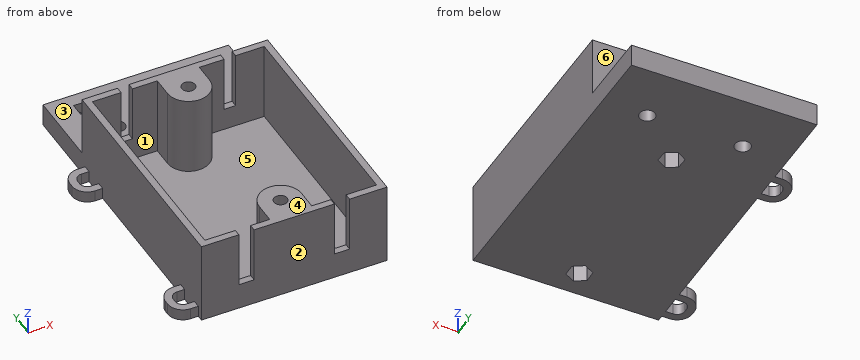
```python
from build123d import *

# Parameters (mm, degrees)
F0_W      = 48.6
F0_H      = 61.2
F1_DEPTH  = 22
F0_R      = 1.75
F2_DEPTH  = 22
F3_DEPTH  = 1
F0_H_2    = 20
F0_R_2    = 2.05
F4_DEPTH  = 6
F5_W      = 3
F5_H      = 1.8
F5_W_2    = 4
F6_DEPTH  = 15
F8_DEPTH  = 7
F9_DEPTH  = 3.5
F11_DEPTH = 5.2
F12_DEPTH = 5
F14_DEPTH = 3


with BuildPart() as f1:
    # F0 (on Top) → F1 (new body)
    with BuildSketch(Plane.XY):
        Rectangle(F0_W, F0_H)
        Polygon((22.5, 28.8), (22.5, -28.8), (5.5, -28.8), (-5.5, -28.8), (-22.5, -28.8), (-22.5, 28.8), (-5.5, 28.8), (5.5, 28.8), align=None, mode=Mode.SUBTRACT)
    extrude(amount=F1_DEPTH)

    # F0 (on Top) → F2 (join)
    with BuildSketch(Plane.XY):
        with BuildLine():
            Line((-5.5, -28.8), (5.5, -28.8))
            Line((5.5, -28.8), (5.5, -23.6))
            ThreePointArc((5.5, -23.6), (0, -18.1), (-5.5, -23.6))
            Line((-5.5, -23.6), (-5.5, -28.8))
        make_face()
        with Locations((0, -23.6)):
            Circle(F0_R, mode=Mode.SUBTRACT)
        with BuildLine():
            Line((5.5, 23.6), (5.5, 28.8))
            Line((5.5, 28.8), (-5.5, 28.8))
            Line((-5.5, 28.8), (-5.5, 23.6))
            ThreePointArc((-5.5, 23.6), (0, 18.1), (5.5, 23.6))
        make_face()
        with Locations((0, 23.6)):
            Circle(F0_R, mode=Mode.SUBTRACT)
    extrude(amount=F2_DEPTH)

    # F0 (on Top) → F3 (join)
    with BuildSketch(Plane.XY):
        with BuildLine():
            Line((5.5, -28.8), (22.5, -28.8))
            Line((22.5, -28.8), (22.5, 28.8))
            Line((22.5, 28.8), (5.5, 28.8))
            Line((5.5, 28.8), (5.5, 23.6))
            ThreePointArc((5.5, 23.6), (0, 18.1), (-5.5, 23.6))
            Line((-5.5, 23.6), (-5.5, 28.8))
            Line((-5.5, 28.8), (-22.5, 28.8))
            Line((-22.5, 28.8), (-22.5, -28.8))
            Line((-22.5, -28.8), (-5.5, -28.8))
            Line((-5.5, -28.8), (-5.5, -23.6))
            ThreePointArc((-5.5, -23.6), (0, -18.1), (5.5, -23.6))
            Line((5.5, -23.6), (5.5, -28.8))
        make_face()
    extrude(amount=F3_DEPTH)

    # F0 (on Top) → F4 (join)
    with BuildSketch(Plane.XY):
        with Locations((0, 40.6)):
            Rectangle(F0_W, F0_H_2)
        with Locations((-12.5, 35.6)):
            Circle(F0_R_2, mode=Mode.SUBTRACT)
        with Locations((12.5, 35.6)):
            Circle(F0_R_2, mode=Mode.SUBTRACT)
    extrude(amount=F4_DEPTH)

    # F5 (on face) → F6 (cut)
    with BuildSketch(Plane.XY.offset(22)):
        with Locations((-13.5, 29.7)):
            Rectangle(F5_W, F5_H)
        with Locations((13.5, 29.7)):
            Rectangle(F5_W, F5_H)
        with Locations((-12.5, -29.7)):
            Rectangle(F5_W_2, F5_H)
        with Locations((12.5, -29.7)):
            Rectangle(F5_W_2, F5_H)
    extrude(amount=-F6_DEPTH, mode=Mode.SUBTRACT)

    # F7 (on face) → F8 (cut)
    with BuildSketch(Plane(origin=(0, 50.6, 0), x_dir=(-1, 0, 0), z_dir=(0, 1, 0))):
        with BuildLine():
            Line((11, 6), (8.9152066989, 6))
            ThreePointArc((8.9152066989, 6), (13.5, 2.3074175964), (18.0847933011, 6))
            Line((18.0847933011, 6), (16, 6))
            ThreePointArc((16, 6), (13.5, 4.3074175964), (11, 6))
        make_face()
        with BuildLine():
            Line((-16, 6), (-18.0847933011, 6))
            ThreePointArc((-18.0847933011, 6), (-13.5, 2.3074175964), (-8.9152066989, 6))
            Line((-8.9152066989, 6), (-11, 6))
            ThreePointArc((-11, 6), (-13.5, 4.3074175964), (-16, 6))
        make_face()
    extrude(amount=-F8_DEPTH, mode=Mode.SUBTRACT)

    # F7 (on face) → F9 (join)
    with BuildSketch(Plane(origin=(0, 50.6, 0), x_dir=(-1, 0, 0), z_dir=(0, 1, 0))):
        with BuildLine():
            Line((11, 6), (8.9152066989, 6))
            ThreePointArc((8.9152066989, 6), (13.5, 2.3074175964), (18.0847933011, 6))
            Line((18.0847933011, 6), (16, 6))
            ThreePointArc((16, 6), (13.5, 4.3074175964), (11, 6))
        make_face()
        with BuildLine():
            Line((-16, 6), (-18.0847933011, 6))
            ThreePointArc((-18.0847933011, 6), (-13.5, 2.3074175964), (-8.9152066989, 6))
            Line((-8.9152066989, 6), (-11, 6))
            ThreePointArc((-11, 6), (-13.5, 4.3074175964), (-16, 6))
        make_face()
    extrude(amount=-F9_DEPTH)

    # F0 (on Top) → F11 (join)
    with BuildSketch(Plane.XY):
        with Locations((0, 23.6)):
            Circle(F0_R)
        with Locations((0, -23.6)):
            Circle(F0_R)
    extrude(amount=F11_DEPTH)

    # F10 (on face) → F12 (cut)
    with BuildSketch(Plane.XY):
        Polygon((-2.7033752158, 21.9341381282), (0.0909910922, 20.4258774513), (2.7943663081, 22.091739323), (2.7033752158, 25.2658618718), (-0.0909910922, 26.7741225487), (-2.7943663081, 25.108260677), align=None)
        Polygon((2.7033752158, -25.2658618718), (2.7943663081, -22.091739323), (0.0909910922, -20.4258774513), (-2.7033752158, -21.9341381282), (-2.7943663081, -25.108260677), (-0.0909910922, -26.7741225487), align=None)
    extrude(amount=F12_DEPTH, mode=Mode.SUBTRACT)

    # F13 (on face) → F14 (join)
    with BuildSketch(Plane.XY):
        with BuildLine():
            Line((-26.3, -29), (-24.3, -29))
            Line((-24.3, -29), (-24.3, -27))
            Line((-24.3, -27), (-26.3, -27))
            ThreePointArc((-26.3, -27), (-27.7142135624, -26.4142135624), (-28.3, -25))
            Line((-28.3, -25), (-28.3, -24))
            ThreePointArc((-28.3, -24), (-27.7142135624, -22.5857864376), (-26.3, -22))
            Line((-26.3, -22), (-24.3, -22))
            Line((-24.3, -22), (-24.3, -20))
            Line((-24.3, -20), (-26.3, -20))
            ThreePointArc((-26.3, -20), (-29.1284271247, -21.1715728753), (-30.3, -24))
            Line((-30.3, -24), (-30.3, -25))
            ThreePointArc((-30.3, -25), (-29.1284271247, -27.8284271247), (-26.3, -29))
        make_face()
        with BuildLine():
            Line((-26.3, 20), (-24.3, 20))
            Line((-24.3, 20), (-24.3, 22))
            Line((-24.3, 22), (-26.3, 22))
            ThreePointArc((-26.3, 22), (-27.7142135624, 22.5857864376), (-28.3, 24))
            Line((-28.3, 24), (-28.3, 25))
            ThreePointArc((-28.3, 25), (-27.7142135624, 26.4142135624), (-26.3, 27))
            Line((-26.3, 27), (-24.3, 27))
            Line((-24.3, 27), (-24.3, 29))
            Line((-24.3, 29), (-26.3, 29))
            ThreePointArc((-26.3, 29), (-29.1284271247, 27.8284271247), (-30.3, 25))
            Line((-30.3, 25), (-30.3, 24))
            ThreePointArc((-30.3, 24), (-29.1284271247, 21.1715728753), (-26.3, 20))
        make_face()
    extrude(amount=F14_DEPTH)


solid = f1.part
```
Could you check a few things on this model? Use its own coordinates, in mm. Face numbers are marked on the shaded views. A direction names the side the tool comes from. Coordinates: 2 decimals unless noted, no trailing zeros. Write each loop counter-clockwise with the first axis right and the second up, starting at its lowest first coordinate (ties: lowest second). Pieces come first, ordered by that corner, then holes. Notation, with made-up numbers: M 56,63.5 L 72,63.5 A19 ccw 72,67.5 Z; hole C 7,-32 d1. An arc over 180 degrees is marked long. Answer as CSV lines item,"result". Start each with the question number.
1) I want a section at A-A, the plane z = 15.5. Give the number of separate pieces and of enclosed holes in the cut face, and give its area (3 significant figures).
2) I want a section at C-C, the plane x = 20. Please give me the cut outline in (y, z), and give its area (3 significant figures).
3) We'd pull the mould along Y, two halves only. Please class the marked faces 1, 2 and 3: +Y half, -Y half, draft (parallel to the pull), parting line (faces both ways), or undercut.
4) For P1, Ø0.6, axis at x = -25, z = 1, coming from the -Y side; P2, Ø5, axis at x = 18.5, z = 13.5, coming from the +Y side; P3, Ø0.5, axis at x = -13.5, y = -30, coming from the +Z side, each with a flat end and sliding along its axis, tell me the tip position at first contact or that it passes through.
5) I want a section at B-B, the plane y = 15. Please give me the cut outline in (x, z).
6) Please list where these lines run through material, in increasing order: line 1 (Y direction, x = 0, z = 18); line 2 (Y direction, x = 12.5, z = 4.6); line 3 (Y direction, x = -12.5, z = 2.6). Write a range as from..to.
7) I want a section at D-D, the plane x = -4. Please give me the cut outline in (y, z).
8) For the marked faces 4, 5 and 6, which set-ups out of +Z, -Z, +X, -X, +Y, -Y let a thin tool reach every point of the face, with its end or its side?
Data:
1,separate pieces,"4"
1,enclosed holes,"2"
1,area,"547 mm^2"
2,outline,"M -30.6,0 L 50.6,0 L 50.6,6 L 30.6,6 L 30.6,22 L 28.8,22 L 28.8,1 L -28.8,1 L -28.8,22 L -30.6,22 Z"
2,area,"257 mm^2"
3,face 1,"undercut"
3,face 2,"-Y half"
3,face 3,"draft"
4,P1,"stops at y = -29"
4,P2,"stops at y = 30.6"
4,P3,"stops at z = 7"
5,outline,"M -24.3,0 L 24.3,0 L 24.3,22 L 22.5,22 L 22.5,1 L -22.5,1 L -22.5,22 L -24.3,22 Z"
6,line 1,"y = -30.6..-25.35, -21.85..-18.1, 18.1..21.85, 25.35..30.6"
6,line 2,"y = -30.6..-28.8, 28.8..33.55, 37.65..50.6"
6,line 3,"y = -30.6..-28.8, 28.8..33.55, 37.65..43.6, 47.1..50.6"
7,outline,"M -30.6,0 L 50.6,0 L 50.6,6 L 30.6,6 L 30.6,22 L 19.83,22 L 19.83,1 L -19.83,1 L -19.83,22 L -30.6,22 Z"
8,face 4,"+Z, +X, -X, +Y, -Y"
8,face 5,"+Z"
8,face 6,"+Z, +X, -X, +Y"
